Source: CAD feature listing. Evaluate the final solid. Frame: model axes, mm. A direction names the side the tool comes from. Give positions to 0.01 mm unless a question says otherwise; leave off trailing zeros. Order: outer loops, then holes, each group sorted by start corner. A loop starts at its lowest first (then second) coordinate and runs counter-clockwise, first axis right, second up. Notation, with made-up numbers: (66, 19.25) - (119, 19.25) arc R29 ccw to (119, 54.25) - close; hole circle Ø5 at (47, 17.25). An arc over 180 degrees is marked (long way). Answer as CSV lines item,"result".
```python
from build123d import *

# Parameters (mm, degrees)
F0_R     = 1.55
F1_DEPTH = 2


# Not quite as in the source:
# - ends of sketch curves that miss each other by under 0.0002 mm in the source are joined


with BuildPart() as f1:
    # F0 (on Top) → F1 (new body)
    with BuildSketch(Plane.XY):
        with BuildLine():
            Line((24.1317584196, 12.0030992724), (24.1317584196, 33.0030992724))
            ThreePointArc((24.1317584196, 33.0030992724), (22.8094861976, 36.1735119864), (19.6355297082, 37.4872550396))
            Line((19.6355297082, 37.4872550396), (-3.1620066842, 37.5062195601))
            ThreePointArc((-3.1620066842, 37.5062195601), (-9.952633868, 35.7733094648), (-15.054516581, 30.9684798394))
            Line((-15.054516581, 30.9684798394), (-21.4377415602, 20.8777601542))
            ThreePointArc((-21.4377415602, 20.8777601542), (-22.515185711, 19.6558592058), (-23.9282391339, 18.8451756363))
            Line((-23.9282391339, 18.8451756363), (-46.5253097099, 10.4110515716))
            ThreePointArc((-46.5253097099, 10.4110515716), (-47.6965598622, 9.7014043841), (-48.3182136925, 8.4811697487))
            Line((-48.3182136925, 8.4811697487), (-48.3182136925, -8.4811697487))
            ThreePointArc((-48.3182136925, -8.4811697487), (-47.6965598622, -9.7014043841), (-46.5253097099, -10.4110515716))
            Line((-46.5253097099, -10.4110515716), (-23.9282391339, -18.8451756363))
            ThreePointArc((-23.9282391339, -18.8451756363), (-22.515185711, -19.6558592058), (-21.4377415602, -20.8777601542))
            Line((-21.4377415602, -20.8777601542), (-15.054516581, -30.9684798394))
            ThreePointArc((-15.054516581, -30.9684798394), (-9.952633868, -35.7733094648), (-3.1620066842, -37.5062195601))
            Line((-3.1620066842, -37.5062195601), (19.6355018203, -37.4872550628))
            ThreePointArc((19.6355018203, -37.4872550628), (22.8150621518, -36.1679133678), (24.1317584196, -32.9872566198))
            Line((24.1317584196, -32.9872566198), (24.1317584196, -12.0030992724))
            Line((24.1317584196, -12.0030992724), (24.1317584196, -12))
            ThreePointArc((24.1317584196, -12), (25.8891177325, -7.7573593129), (30.1317584196, -6))
            Line((30.1317584196, -6), (36.1317584196, -6))
            ThreePointArc((36.1317584196, -6), (40.3733032071, -4.2437363038), (42.1317576192, -0.003099272))
            Line((42.1317576192, -0.003099272), (42.1317584196, 0))
            ThreePointArc((42.1317584196, 0), (40.3743991067, 4.2426406871), (36.1317584196, 6))
            Line((36.1317584196, 6), (30.1317584196, 6))
            ThreePointArc((30.1317584196, 6), (25.8891177325, 7.7573593129), (24.1317584196, 12))
            Line((24.1317584196, 12), (24.1317584196, 12.0030992724))
        make_face()
        with Locations((-44.3682136925, -7)):
            Circle(F0_R, mode=Mode.SUBTRACT)
        with Locations((12.6317863075, -32.9930796663)):
            Circle(F0_R, mode=Mode.SUBTRACT)
        with Locations((19.1317584196, -25)):
            Circle(F0_R, mode=Mode.SUBTRACT)
        with Locations((19.6317863075, -32.9872565966)):
            Circle(F0_R, mode=Mode.SUBTRACT)
        with Locations((-44.3682136925, 7)):
            Circle(F0_R, mode=Mode.SUBTRACT)
        with BuildLine():
            Line((-14.2339508783, 15.4306240067), (-7.4342503505, 26.1797159146))
            ThreePointArc((-7.4342503505, 26.1797159146), (-5.5889861734, 27.9038009834), (-3.1365199939, 28.5061952445))
            Line((-3.1365199939, 28.5061952445), (8.1350859734, 28.4968187664))
            ThreePointArc((8.1350859734, 28.4968187664), (10.9616557954, 27.323776346), (12.1317584196, 24.4959882833))
            Line((12.1317584196, 24.4959882833), (12.1317584196, -24.4985477622))
            ThreePointArc((12.1317584196, -24.4985477622), (10.9611450551, -27.3260150506), (8.1344727862, -28.4985468413))
            Line((8.1344727862, -28.4985468413), (-3.1365199939, -28.5061952445))
            ThreePointArc((-3.1365199939, -28.5061952445), (-5.5889861734, -27.9038009834), (-7.4342503505, -26.1797159146))
            Line((-7.4342503505, -26.1797159146), (-14.2339508783, -15.4306240067))
            ThreePointArc((-14.2339508783, -15.4306240067), (-15.0416860208, -13.6364803831), (-15.3182136925, -11.688424981))
            Line((-15.3182136925, -11.688424981), (-15.3182136925, 11.688424981))
            ThreePointArc((-15.3182136925, 11.688424981), (-15.0416860208, 13.6364803831), (-14.2339508783, 15.4306240067))
        make_face(mode=Mode.SUBTRACT)
        with Locations((36.1317584196, 0)):
            Circle(F0_R, mode=Mode.SUBTRACT)
        with Locations((19.1317584196, 25)):
            Circle(F0_R, mode=Mode.SUBTRACT)
        with Locations((12.6317863075, 32.9930796663)):
            Circle(F0_R, mode=Mode.SUBTRACT)
        with Locations((19.6317863075, 32.9872565966)):
            Circle(F0_R, mode=Mode.SUBTRACT)
    extrude(amount=F1_DEPTH)


solid = f1.part
```
(1) Cut plane A-A (y = -7). Return loops of the section in (x, z), then the cut area to 3 significant figures.
Completed:
outline,"(-48.32, 0) - (-45.92, 0) - (-45.92, 2) - (-48.32, 2) - close; (-42.82, 0) - (-15.32, 0) - (-15.32, 2) - (-42.82, 2) - close; (12.13, 0) - (26.82, 0) - (26.82, 2) - (12.13, 2) - close"
area,"89.2 mm²"
(2) Cut plane C-C (z = 1.05). Give the number of separate pieces and of enclosed holes in the cut face, then the cut area to 3 significant figures.
Completed:
separate pieces,"1"
enclosed holes,"10"
area,"2,740 mm²"
(3) Ray query, line 1 (X direction, y = -24.5, z = 1.6); line 2 (X direction, y = 1, z = 0.8); line 3 (Y direction, x = 30, z = 1). Return the intervals inside material, ascending. Write a range as from..to.
Completed:
line 1,"-19.15..-8.5, 12.13..17.66, 20.6..24.13"
line 2,"-48.32..-15.32, 12.13..34.95, 37.32..42.05"
line 3,"-6..6"
(4) Contact query for flat-ended pins moving along their axis: pin 1 (1 mm diameter, centred on x = -27, z = 1.5, fed in from +Y); pin 2 (0.6 mm diameter, centred on x = 33, z = 1, fed in from +Y); pin 3 (1 mm diameter, centred on x = 10.5, z = 1, fed in from +Y). Output: stop coordinate, or through.
Completed:
pin 1,"y = 17.89"
pin 2,"y = 6"
pin 3,"y = 37.5"
(5) Cut plane D-D (x = -25.5). Return loops of the section in (y, z).
Completed:
outline,"(-18.26, 0) - (18.26, 0) - (18.26, 2) - (-18.26, 2) - close"
(6) Access query for faces 5 (the cylindrical face through (-47.7, -9.7, 1)), 6 (the flat face through (-10.9, 20.7, 1)), 7 (the flat face through (33, 6, 1)). Directions: +Z, -Z, +X, -X, +Y, -Y. A direction counts if a zero-diameter tool reaches every point of the face in a straight line with its end or side. Return the directions, or none.
Completed:
face 5,"+Z, -Z, -X, -Y"
face 6,"+Z, -Z"
face 7,"+Z, -Z, +X, +Y"
(7) Mould query, pull axis Y, two halves, no side actions, for faces 1 (the cylindrical face through (40.326, -4.29, 0.986)), 2 (the cylindrical face through (37.6, 0.5, 1)), 3 (the flat face through (24.132, 22, 1)), 4 (the cylindrical face through (-5.6, -27.9, 1)). Classes: released by +Y, released by -Y, zero draft, split by the parting line, or undercut.
Completed:
face 1,"released by -Y"
face 2,"undercut"
face 3,"zero draft"
face 4,"undercut"
(8) Cut plane B-B (y = -27.5). Return loops of the section in (x, z), then the cut area to 3 significant figures.
Completed:
outline,"(-17.25, 0) - (-6.22, 0) - (-6.22, 2) - (-17.25, 2) - close; (10.78, 0) - (24.13, 0) - (24.13, 2) - (10.78, 2) - close"
area,"48.8 mm²"
